The model under review builds one solid part; all positions refer to its coordinate system, in mm. Face numbers are marked on the shaded views. A direction names the side the tool comes from. Coordinates: 2 decimals unless noted, no trailing zeros. Loops run counter-clockwise (first coordinate to the right, second up) from the corner with the lowest first, then second, coordinate; pieces in that order, holes last. Notation, with made-up numbers: M 1.25,78.5 L 27.25,78.5 A13 cw 27.25,94.5 Z; hole C 71.5,20.5 d3. An arc over 180 degrees is marked long. Use CSV: the item, a comma, the result in double quotes. Start each with the question number.
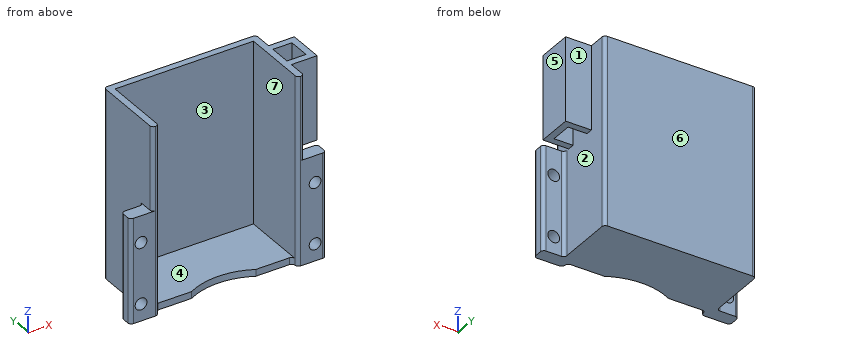
from build123d import *

# Parameters (mm, degrees)
BOSS_EXTRUDE1_DEPTH = 70.612
SKETCH2_R           = 2.2
CUT_EXTRUDE1_DEPTH  = 83.799422419
SKETCH3_W           = 8.255
SKETCH3_H           = 31.401404102
CUT_EXTRUDE2_DEPTH  = 83.799422419
BOSS_EXTRUDE3_DEPTH = 2.54
CUT_EXTRUDE6_DEPTH  = 2.54
SKETCH9_W           = 51.816
SKETCH9_H           = 2.54
CUT_EXTRUDE7_DEPTH  = 2.54
FILLET1_R           = 1.27
FILLET2_R           = 1.27
BOSS_EXTRUDE4_DEPTH = 31.401404102


with BuildPart() as part:
    # Sketch1 → Boss-Extrude1 (new body)
    with BuildSketch(Plane.XY):
        Polygon((25.908, 25.4), (-25.908, 25.4), (-25.908, 0), (-36.703, 0), (-36.703, 5.08), (-28.448, 5.08), (-28.448, 27.94), (28.448, 27.94), (28.448, 5.08), (36.703, 5.08), (36.703, 0), (25.908, 0), align=None)
    extrude(amount=BOSS_EXTRUDE1_DEPTH)

    # Sketch2 → Cut-Extrude1 (cut, through all)
    with BuildSketch(Plane(origin=(0, 5.08, 0), x_dir=(1, 0, 0), z_dir=(0, 1, 0))):
        with Locations(Location((-32.5755, -6.35, 0), (0, 0, 270))):
            Circle(SKETCH2_R)
        with Locations(Location((-32.5755, -29.21, 0), (0, 0, 270))):
            Circle(SKETCH2_R)
    cut_extrude1 = extrude(amount=-CUT_EXTRUDE1_DEPTH, mode=Mode.SUBTRACT)

    # Mirror1: Cut-Extrude1 across plane
    add(cut_extrude1.mirror(Plane(origin=(0, 0, 0), x_dir=(0, 0, 1), z_dir=(1, 0, 0))), mode=Mode.SUBTRACT)

    # Sketch3 → Cut-Extrude2 (cut, through all)
    with BuildSketch(Plane(origin=(0, 5.08, 0), x_dir=(1, 0, 0), z_dir=(0, 1, 0))):
        with Locations((-32.5755, -54.911297949)):
            Rectangle(SKETCH3_W, SKETCH3_H)
        with Locations((32.5755, -54.911297949)):
            Rectangle(SKETCH3_W, SKETCH3_H)
    extrude(amount=-CUT_EXTRUDE2_DEPTH, mode=Mode.SUBTRACT)

    # Sketch6 → Boss-Extrude3 (add)
    with BuildSketch(Plane(origin=(0, 0, 0), x_dir=(-1, 0, 0), z_dir=(0, 0, -1))):
        Polygon((-25.908, 0), (25.908, 0), (36.703, 0), (36.703, 5.08), (28.448, 5.08), (28.448, 27.94), (-28.448, 27.94), (-28.448, 5.08), (-36.703, 5.08), (-36.703, 0), align=None)
    extrude(amount=-BOSS_EXTRUDE3_DEPTH)

    # Sketch8 → Cut-Extrude6 (cut)
    with BuildSketch(Plane(origin=(0, 0, 0), x_dir=(-1, 0, 0), z_dir=(0, 0, -1))):
        with BuildLine():
            Line((-15.875, 0), (15.875, 0))
            ThreePointArc((15.875, 0), (0, 5.572131355), (-15.875, 0))
        make_face()
    extrude(amount=-CUT_EXTRUDE6_DEPTH, mode=Mode.SUBTRACT)

    # Sketch9 → Cut-Extrude7 (cut)
    with BuildSketch(Plane(origin=(0, 0, 0), x_dir=(-1, 0, 0), z_dir=(0, 0, -1))):
        with Locations((0, 1.27)):
            Rectangle(SKETCH9_W, SKETCH9_H)
    extrude(amount=-CUT_EXTRUDE7_DEPTH, mode=Mode.SUBTRACT)

    # Fillet1
    fillet1_edges = [part.edges().sort_by_distance(p)[0] for p in [
        (-28.448, 5.08, 19.605297949),
        (28.448, 5.08, 19.605297949),
        (36.703, 0, 19.605297949),
        (36.703, 5.08, 19.605297949),
        (-36.703, 5.08, 19.605297949),
        (-36.703, 0, 19.605297949),
        (28.448, 0, 54.911297949),
        (25.908, 0, 35.306),
        (-25.908, 0, 35.306),
        (-28.448, 0, 54.911297949),
        (28.448, 27.94, 35.306),
        (-28.448, 27.94, 35.306),
    ]]
    fillet(fillet1_edges, radius=FILLET1_R - 0.0001)  # a hair under: the kernel refuses the full size

    # Fillet2
    fillet2_edges = [part.edges().sort_by_distance(p)[0] for p in [
        (-25.908, 2.54, 1.27),
        (25.908, 2.54, 1.27),
    ]]
    fillet(fillet2_edges, radius=FILLET2_R)

    # Sketch10 → Boss-Extrude4 (add)
    with BuildSketch(Plane.XY.offset(70.612)):
        Polygon((28.448, 20.574), (38.1, 20.574), (38.1, 7.366), (28.448, 7.366), (28.448, 9.906), (35.56, 9.906), (35.56, 18.034), (28.448, 18.034), align=None)
    extrude(amount=-BOSS_EXTRUDE4_DEPTH)


solid = part.part
1. Insertion check: pin 1 Ø2 at (y, z) = (23, 44.5) entering from +X; pin 2 Ø4 at (x, y) = (6, 7.5) entering from +Z; pin 3 Ø5 at (x, z) = (35.5, 52) entering from -Y; pin 4 Ø10 at (x, y) = (2.5, 5) entering from -Z. Each pin has a flat end and moves straight along its axis. Give the tip position at first contact, or say it passes through.
2. Add section D-D (x = 18.5). Write out the cut boundary in (y, z), plus the area to 3 significant figures.
3. For the marked faces 1, 2 and 3, list the 3-axis set-ups (+Z, -Z, +X, -X, +Y, -Y) from which the entire face can be reached by the end or side of a thin tool; tool diameter is ignored.
4. To check wall thickness, follow line 1 along X through (y, z) = (3.2, 6.35); line 2 along Y through (x, z) = (31, 53.5); line 3 along X through (y, z) = (5.25, 47). State the ranges of each line that lie inside material, in increasing order.
5. Draft analysis for pull direction X (two halves, no side actions). For the marked faces 4, 5, 6 and 7, state which applies: released by +X, released by -X, zero draft, split by the parting line, or undercut.
6. Add section C-C (y = 14.5). Write out the cut boundary in (x, z), plus the area to 3 significant figures.
7. Add section A-A (z = 29.21). Give the number of separate pieces and of enclosed holes in the cut face, plus the area to 3 significant figures.
Solved:
1,pin 1,"stops at x = 28.45"
1,pin 2,"stops at z = 2.54"
1,pin 3,"stops at y = 7.37"
1,pin 4,"stops at z = 0"
2,outline,"M 2.54,0 L 27.94,0 L 27.94,70.61 L 25.4,70.61 L 25.4,2.54 L 2.54,2.54 Z"
2,area,"237 mm^2"
3,face 1,"+Z, -Z, +X, +Y"
3,face 2,"none"
3,face 3,"+Z, -Y"
4,line 1,"x = -36.7 to -34.78, -30.38 to -25.91, 25.91 to 30.38, 34.78 to 36.7"
4,line 2,"y = 7.37 to 9.91, 18.03 to 20.57"
4,line 3,"x = -28.45 to -25.91, 25.91 to 28.45"
5,face 4,"undercut"
5,face 5,"released by +X"
5,face 6,"zero draft"
5,face 7,"undercut"
6,outline,"M -28.45,0 L 28.45,0 L 28.45,70.61 L 25.91,70.61 L 25.91,2.54 L -25.91,2.54 L -25.91,70.61 L -28.45,70.61 Z; M 35.56,39.21 L 38.1,39.21 L 38.1,70.61 L 35.56,70.61 Z"
6,area,"570 mm^2"
7,separate pieces,"3"
7,enclosed holes,"0"
7,area,"311 mm^2"
